Geometry check sheet. Reference: the model listing, model coordinates, mm. A direction names the side the tool comes from. Coordinates: 2 decimals unless noted, no trailing zeros. Loops run counter-clockwise (first coordinate to the right, second up) from the corner with the lowest first, then second, coordinate; pieces in that order, holes last.
from build123d import *

# Parameters (mm, degrees)
BOSS_EXTRUDE2_DEPTH     = 38.1
CUT_EXTRUDE1_DEPTH      = 46.800854849
CUT_EXTRUDE1_DEPTH_BACK = 46.800854849
SKETCH2_R               = 4.445
CUT_EXTRUDE3_DEPTH      = 47.878313216
CUT_EXTRUDE3_DEPTH_BACK = 47.878313216
SKETCH3_R               = 3.302


with BuildPart() as part:
    # Sketch1 → Boss-Extrude2 (new body)
    with BuildSketch(Plane.XY):
        Polygon((-5.548232323, 15.875), (-5.548232323, -3.175), (19.851767677, -3.175), (19.851767677, 0), (-2.373232323, 0), (-2.373232323, 15.875), align=None)
    extrude(amount=BOSS_EXTRUDE2_DEPTH)

    # Sketch2 → Cut-Extrude1 (cut, two sides: drawn at the far end of the back side and taken through both)
    with BuildSketch(Plane(origin=(0, 0, 0), x_dir=(1, 0, 0), z_dir=(0, 1, 0)).offset(-CUT_EXTRUDE1_DEPTH_BACK)):
        with Locations(Location((10.326767677, -19.078550513, 0), (0, 0, 180))):
            Circle(SKETCH2_R)
    extrude(amount=CUT_EXTRUDE1_DEPTH + CUT_EXTRUDE1_DEPTH_BACK, mode=Mode.SUBTRACT)

    # Sketch3 → Cut-Extrude3 (cut, two sides: drawn at the far end of the back side and taken through both)
    with BuildSketch(Plane(origin=(-2.373232323, 0, 0), x_dir=(0, 0, -1), z_dir=(1, 0, 0)).offset(-CUT_EXTRUDE3_DEPTH_BACK)):
        with Locations(Location((-6.269326955, 7.9375, 0), (0, 0, 90))):
            Circle(SKETCH3_R)
        with Locations(Location((-31.669326955, 7.9375, 0), (0, 0, 90))):
            Circle(SKETCH3_R)
    extrude(amount=CUT_EXTRUDE3_DEPTH + CUT_EXTRUDE3_DEPTH_BACK, mode=Mode.SUBTRACT)


solid = part.part
1) Mould release check, pull along Y, two halves, no side actions. Record for faces 3 (the flat face through (-4, 15.875, 19)), 4 (the flat face through (-5.548, 6, 19)), 5 (the cylindrical face through (-3.983, 11.087, 32.661)): +Y half, -Y half, draft (parallel to the pull), parting line (faces both ways), or undercut.
Data:
face 3: +Y half
face 4: draft
face 5: undercut
2) Section check B-B on y = 8.25. Record the cut outline in (x, z).
Data:
outline: (-5.55, 0) - (-2.37, 0) - (-2.37, 2.98) - (-5.55, 2.98) - close; (-5.55, 9.56) - (-2.37, 9.56) - (-2.37, 28.38) - (-5.55, 28.38) - close; (-5.55, 34.96) - (-2.37, 34.96) - (-2.37, 38.1) - (-5.55, 38.1) - close
3) Material ranges on probe 1 along Y at (x, z) = (1.5, 27.5) (3 decimals); probe 2 along X at (y, z) = (4.75, 19), recorded low to high.
Data:
probe 1: y = -3.175 to 0
probe 2: x = -5.55 to -2.37
4) Access from +Z, -Z, +X, -X, +Y, -Y to the whole of each face (thin tool, end or side, straight path). Record for faces 1 (the flat face through (-2.373, 8, 19)), 2 (the flat face through (19.852, -2, 19)).
Data:
face 1: +Z, -Z, +X, +Y
face 2: +Z, -Z, +X, +Y, -Y
5) Section check C-C on x = 11. Record the cut outline in (y, z) (3 decimals).
Data:
outline: (-3.175, 0) - (0, 0) - (0, 14.685) - (-3.175, 14.685) - close; (-3.175, 23.472) - (0, 23.472) - (0, 38.1) - (-3.175, 38.1) - close
6) Section check A-A on z = 31. Record the cut outline in (x, y) (3 decimals).
Data:
outline: (-5.548, -3.175) - (19.852, -3.175) - (19.852, 0) - (-2.373, 0) - (-2.373, 4.704) - (-5.548, 4.704) - close; (-5.548, 11.171) - (-2.373, 11.171) - (-2.373, 15.875) - (-5.548, 15.875) - close
7) Section check D-D on z = 35.5. Record the cut outline in (x, y) (3 decimals).
Data:
outline: (-5.548, -3.175) - (19.852, -3.175) - (19.852, 0) - (-2.373, 0) - (-2.373, 15.875) - (-5.548, 15.875) - close
8) Depth check by flat-ended pin: pin 1 (4 mm diameter, centred on x = 10.5, z = 26.5, fed in from +Y); pin 2 (10 mm diameter, centred on x = 3, y = 3, fed in from -Z); pin 3 (1 mm diameter, centred on y = 12.5, z = 11, fed in from +X). Enter the tip coordinate at first touch or a pass-through.
Data:
pin 1: stops at y = 0
pin 2: stops at z = 0
pin 3: stops at x = -2.37
